```python
from build123d import *

# Parameters (mm, degrees)
SKETCH1_W           = 203.2
SKETCH1_H           = 254
BOSS_EXTRUDE1_DEPTH = 5.08
FILLET1_SIZE        = 59.266666667
FILLET1_SIZE_2      = 101.6
SKETCH7_W           = 5.08
SKETCH7_H           = 50.8
CUT_EXTRUDE1_DEPTH  = 326.318377121


with BuildPart() as part:
    # Sketch1 → Boss-Extrude1 (new body)
    with BuildSketch(Plane.XY):
        with Locations((101.6, 127)):
            Rectangle(SKETCH1_W, SKETCH1_H)
    extrude(amount=BOSS_EXTRUDE1_DEPTH)

    # Fillet1
    # a fillet whose section is not a circle: 101.6, 59.266666667 mm, written as the material it takes off along each edge
    with BuildSketch(Plane(origin=(203.2, 254, -254), x_dir=(0, -1, 0), z_dir=(0, 0, 1))) as fillet1_piece_1:
        with BuildLine():
            Bezier((FILLET1_SIZE, 0), (0, 0), (0, -FILLET1_SIZE_2), weights=[1, 1, 1])
            Line((0, -FILLET1_SIZE_2), (0, 0))
            Line((0, 0), (FILLET1_SIZE, 0))
        make_face()
    extrude(amount=513.08, mode=Mode.SUBTRACT)
    with BuildSketch(Plane(origin=(0, 254, -254), x_dir=(1, 0, 0), z_dir=(0, 0, 1)), Plane(origin=(203.2, 0, -254), x_dir=(-1, 0, 0), z_dir=(0, 0, 1))) as fillet1_piece_2:
        with BuildLine():
            Bezier((FILLET1_SIZE_2, 0), (0, 0), (0, -FILLET1_SIZE), weights=[1, 1, 1])
            Line((0, -FILLET1_SIZE), (0, 0))
            Line((0, 0), (FILLET1_SIZE_2, 0))
        make_face()
    extrude(amount=513.08, mode=Mode.SUBTRACT)
    with BuildSketch(Plane(origin=(0, 0, -254), x_dir=(1, 0, 0), z_dir=(0, 0, 1))) as fillet1_piece_3:
        with BuildLine():
            Bezier((FILLET1_SIZE_2, 0), (0, 0), (0, FILLET1_SIZE), weights=[1, 1, 1])
            Line((0, FILLET1_SIZE), (0, 0))
            Line((0, 0), (FILLET1_SIZE_2, 0))
        make_face()
    extrude(amount=513.08, mode=Mode.SUBTRACT)

    # Sketch7 → Cut-Extrude1 (cut, through all)
    with BuildSketch(Plane.XY.offset(5.08)):
        with Locations((6.096, 169.333333333)):
            Rectangle(SKETCH7_W, SKETCH7_H)
        with Locations((40.894, 169.333333333)):
            Rectangle(SKETCH7_W, SKETCH7_H)
        with Locations((197.104, 169.333333333)):
            Rectangle(SKETCH7_W, SKETCH7_H)
        with Locations((162.306, 169.333333333)):
            Rectangle(SKETCH7_W, SKETCH7_H)
    extrude(amount=-CUT_EXTRUDE1_DEPTH, mode=Mode.SUBTRACT)


solid = part.part
```
For this review, take the finished solid that the model builds, in its own axes (mm). A direction names the side the tool comes from. Coordinates: 2 decimals unless noted, no trailing zeros. Write each loop counter-clockwise with the first axis right and the second up, starting at its lowest first coordinate (ties: lowest second). Pieces come first, ordered by that corner, then holes.
(1) Tool access review of faces 3 (the face through (199.644, 169, 3)), 4 (the face through (0, 126, 3)): name each direction out of +Z, -Z, +X, -X, +Y, -Y from which nothing blocks a thin tool from reaching the whole face with its end or side.
(2) The part is to be moulded in two halves that separate along Y. For faces 1 (the face through (100, 129, 5.08)), 2 (the face through (41, 143.933, 3)), say which applies: +Y half, -Y half, draft (parallel to the pull), parting line (faces both ways), or undercut.
(3) Wall thickness on probe 1 along X at (y, z) = (144, 4.85); probe 2 along Y at (x, z) = (99, 4.6); probe 3 along X at (y, z) = (239, 4.7): over which ranges is each line inside the solid? List them lowest first.
(4) Add section B-B on z = 3.15. Count the separate pieces of the cut face and the enclosed holes in it, then the cut area to 3 significant figures.
(5) For pin 1 Ø2 at (x, z) = (164, 4) entering from -Y; pin 2 Ø2.5 at (x, z) = (41, 1.5) entering from +Y; pin 3 Ø1 at (y, z) = (57, 1.5) entering from -X, all flat-tipped, find the tip position at first contact; note any pin that passes through.
(6) Add section A-A on y = 167. Give the boundary of the cut face in (x, z), then the cut area to 3 significant figures.
Answer sheet:
1. face 3: +Z, -Z
1. face 4: +Z, -Z, -X, +Y, -Y
2. face 1: draft
2. face 2: undercut
3. probe 1: x = 0 to 3.56, 8.64 to 38.35, 43.43 to 159.77, 164.85 to 194.56, 199.64 to 203.2
3. probe 2: y = 0.01 to 253.99
3. probe 3: x = 25.09 to 178.11
4. separate pieces: 1
4. enclosed holes: 4
4. area: 46,600 mm2
5. pin 1: stops at y = 8.16
5. pin 2: stops at y = 246.53
5. pin 3: stops at x = 0.02
6. outline: (0, 0) - (3.56, 0) - (3.56, 5.08) - (0, 5.08) - close; (8.64, 0) - (38.35, 0) - (38.35, 5.08) - (8.64, 5.08) - close; (43.43, 0) - (159.77, 0) - (159.77, 5.08) - (43.43, 5.08) - close; (164.85, 0) - (194.56, 0) - (194.56, 5.08) - (164.85, 5.08) - close; (199.64, 0) - (203.2, 0) - (203.2, 5.08) - (199.64, 5.08) - close
6. area: 929 mm2
